Autodesk Inventor part; units mm, degrees
ref_plane "YZ Plane" through (0, 0, 0) normal (1, 0, 0) x (0, 1, 0)
ref_plane "XZ Plane" through (0, 0, 0) normal (0, 1, 0) x (-1, 0, 0)
ref_plane "XY Plane" through (0, 0, 0) normal (0, 0, 1) x (1, 0, 0)
sketch "Sketch1" plane through (0, 0, 0) normal (0, 0, 1) x (1, 0, 0)
  line L0 (0, 0) -> (0, 152.8559)
  line L1 (0, 152.8559) -> (-25, 138.4222)
  line L2 (-25, 138.4222) -> (-25, 0)
  line L3 (-25, 0) -> (25, 0)
  line L4 (25, 0) -> (25, 138.4222)
  line L5 (25, 138.4222) -> (0, 152.8559)
  dimension "d0" = 152.8559
  dimension "d1" = 60
  dimension "d2" = 60
  dimension "d3" = 50
extrude "Extrusion1" add sketch "Sketch1" along normal blind 10
sketch "Sketch2" plane through (0, 0, 0) normal (0, 0, -1) x (-1, 0, 0)
  line L0 (0, 152.8559) -> (25, 138.4222)
  line L1 (-25, 138.4222) -> (0, 152.8559)
  line L2 (25, 0) -> (-25, 0)
  line L3 (-25, 0) -> (25, 0)
  line L4 (25, 0) -> (25, 10)
  line L5 (25, 10) -> (-25, 10)
  line L6 (-25, 10) -> (-25, 0)
  line L7 (25, 138.4222) -> (25, 0) construction
  line L8 (-25, 0) -> (-25, 138.4222) construction
  line L9 (-25, 126.8751) -> (0, 141.3089)
  line L10 (0, 141.3089) -> (25, 126.8751)
  line L11 (25, 138.4222) -> (25, 0)
  line L12 (-25, 126.8751) -> (-25, 138.4222)
  line L13 (0, 152.8559) -> (25, 138.4222)
  line L14 (25, 126.8751) -> (25, 138.4222)
  point P0 (0, 0)
  dimension "d6" = 10
  dimension "d7" = 10
extrude "Extrusion2" add sketch "Sketch2" along normal blind 50
sketch "Sketch3" plane through (0, 141.3089, -50) normal (-0.5, -0.8660254, 0) x (0.8660254, -0.5, 0)
  circle A0 centre (14.4338, 25) radius 2.5
  line L0 (28.8675, 50) -> (28.8675, 0)
  line L1 (28.8675, 0) -> (0, 0)
  point P0 (70.6545, 50)
  point P1 (14.4338, 0)
  point P2 (28.8675, 25)
  dimension "d10" = 5
extrude "Extrusion3" cut sketch "Sketch3" against normal through all
sketch "Sketch4" plane through (-25, 126.8751, -50) normal (0.5, -0.8660254, 0) x (0.8660254, 0.5, 0)
  line L0 (0, 50) -> (0, 0)
  line L1 (28.8675, 0) -> (0, 0)
  circle A0 centre (14.4338, 25) radius 2.5
  point P0 (-41.7869, 50)
  point P1 (14.4338, 0)
  point P2 (0, 25)
  dimension "d13" = 5
extrude "Extrusion4" cut sketch "Sketch4" against normal through all
sketch "Sketch5" plane through (-25, 10, 0) normal (0, 1, 0) x (1, 0, 0)
  line L0 (0, 0) -> (0, 50)
  line L1 (0, 50) -> (50, 50)
  circle A0 centre (25, 25) radius 2.5
  point P0 (25, 0)
  point P1 (25, 50)
  point P2 (0, 25)
  dimension "d16" = 5
extrude "Extrusion5" cut sketch "Sketch5" against normal through all
sketch "Sketch6" plane through (0, 0, 10) normal (0, 0, 1) x (1, 0, 0)
  circle A0 centre (0, 76.428) radius 6
  line L0 (-25, 138.4222) -> (0, 152.8559) construction
  line L1 (0, 152.8559) -> (0, 0) construction
  circle A1 centre (0, 69.428) radius 1.5 construction
  circle A2 centre (15.5, 69.428) radius 1.5
  circle A3 centre (7.75, 82.8513) radius 1.5
  circle A4 centre (-7.75, 82.8513) radius 1.5
  circle A5 centre (-15.5, 69.428) radius 1.5
  circle A6 centre (-7.75, 56.0046) radius 1.5
  circle A7 centre (7.75, 56.0046) radius 1.5
  point P0 (0, 76.428)
  dimension "d19" = 12
  dimension "d22" = 3
  dimension "d23" = 7
  dimension "d24" = 3
  dimension "d25" = 15.5
  dimension "d28" = 360
extrude "Extrusion6" cut sketch "Sketch6" against normal through all
sketch "Sketch7" plane through (0, 0, 0) normal (0, 0, -1) x (-1, 0, 0)
  circle A0 centre (-7.75, 56.0046) radius 1.5
  circle A1 centre (15.5, 69.428) radius 1.5
  circle A2 centre (-7.75, 82.8513) radius 1.5
  circle A3 centre (-15.5, 69.428) radius 1.5
  circle A4 centre (7.75, 82.8513) radius 1.5
  circle A5 centre (7.75, 56.0046) radius 1.5
  circle A6 centre (0, 76.428) radius 6
  line L0 (-25, 10) -> (25, 10)
  line L1 (25, 126.8751) -> (25, 10)
  line L2 (25, 126.8751) -> (0, 141.3089)
  line L3 (0, 141.3089) -> (-25, 126.8751)
  line L4 (-25, 10) -> (-25, 126.8751)
  circle A7 centre (0, 69.428) radius 20
  point P0 (0, 0)
  dimension "d32" = 40
extrude "Extrusion7" cut sketch "Sketch7" against normal blind 5 contours A0 | A1 | A2 | A3 | A4 | A5 | A6 | A7
sketch "Sketch8" plane through (0, 0, 10) normal (0, 0, 1) x (1, 0, 0)
  circle A0 centre (15.5, 69.428) radius 1.5
  circle A1 centre (0, 69.428) radius 1.5
  line L0 (-25, 0) -> (25, 0)
  circle A2 centre (15.5, 69.428) radius 4
  circle A3 centre (7.75, 82.8513) radius 4
  circle A4 centre (-7.75, 82.8513) radius 4
  circle A5 centre (-15.5, 69.428) radius 4
  circle A6 centre (-7.75, 56.0046) radius 4
  circle A7 centre (7.75, 56.0046) radius 4
  point P0 (0, 0)
  point P1 (0, 0)
  dimension "d35" = 3
  dimension "d36" = 8
  dimension "d39" = 360
extrude "Extrusion8" cut sketch "Sketch8" against normal blind 3 contours A0 | A2 | A3 | A4 | A5 | A6 | A7
properties part number "BO12" material "ABS Plastic"
Can you work these out from the model? Positions are in its coordinate system, mm. A direction names the side the tool comes from. Coordinates: 2 decimals unless noted, no trailing zeros. Order: outer loops, then holes, each group sorted by start corner. A loop starts at its lowest first (then second) coordinate and runs counter-clockwise, first axis right, second up.
1. If we section it at B-B (x = 7.75): Please give me the cut outline in (y, z).
2. If we section it at D-D (z = -25): Please give me the cut outline in (x, y), then the cut area to 3 significant figures.
3. For faces 4 (the face through (-15.6, 67.7, 7)), 5 (the face through (-8.08, 54.54, 6.01)), 6 (the face through (-25, 64, 2)), 7 (the face through (0, 10, -19)), 8 (the face through (-15.1, 132.59, -24.65)), which set-ups out of +Z, -Z, +X, -X, +Y, -Y let a thin tool reach every point of the face, with its end or its side?
4. If we section it at A-A (z = -43.5): Please give me the cut outline in (x, y).
5. I need wall thicknesses on line 1 (Y direction, x = 7, z = 6); line 2 (Z direction, x = -12, y = 108.5); line 3 (Z direction, x = 17, y = 76). Which ranges of each line are inside material? Lowest first, please.
6. I'm going to push flat-ended pins straight in: pin 1 (4 mm diameter, centred on x = 7.75, y = 56, fed in from +Z); pin 2 (7 mm diameter, centred on x = 0, y = 76.428, fed in from -Z); pin 3 (5 mm diameter, centred on x = 15.5, y = 69.428, fed in from -Z); pin 4 (25 mm diameter, centred on x = -11.5, y = 43, fed in from -Z). Where does each tip first touch, or does it pass through?
7. Thinking about a two-plate mould opening in Y: for faces 1 (the face through (-12.325, 145.74, -20.42)), 2 (the face through (0, 0, -20)), 3 (the face through (9.897, 135.595, -24.65)), which applies, +Y half, -Y half, draft (parallel to the pull), parting line (faces both ways), or undercut?
8. If we section it at C-C (y = 17.5): Please give me the cut outline in (x, z), then the cut area to 3 significant figures.
Entries:
1. outline: (0, -50) - (10, -50) - (10, 0) - (50.99, 0) - (50.99, 5) - (54.5, 5) - (54.5, 7) - (52, 7) - (52, 10) - (0, 10) - close; (57.5, 5) - (81.35, 5) - (81.35, 7) - (78.85, 7) - (78.85, 10) - (60, 10) - (60, 7) - (57.5, 7) - close; (84.35, 5) - (87.87, 5) - (87.87, 0) - (136.83, 0) - (136.83, -50) - (148.38, -50) - (148.38, 10) - (86.85, 10) - (86.85, 7) - (84.35, 7) - close
2. outline: (-25, 0) - (-2.5, 0) - (-2.5, 10) - (-25, 10) - close; (-25, 126.88) - (-14.67, 132.84) - (-19.67, 141.5) - (-25, 138.42) - close; (-15.33, 144) - (-10.33, 135.34) - (0, 141.31) - (10.33, 135.34) - (15.33, 144) - (0, 152.86) - close; (2.5, 0) - (25, 0) - (25, 10) - (2.5, 10) - close; (14.67, 132.84) - (25, 126.88) - (25, 138.42) - (19.67, 141.5) - close
2. area: 927 mm2
3. face 4: +Z
3. face 5: +Z, -Z
3. face 6: +Z, -Z, -X, +Y, -Y
3. face 7: -Z, +X, -X
3. face 8: -Z
4. outline: (-25, 0) - (25, 0) - (25, 10) - (-25, 10) - close; (-25, 126.88) - (0, 141.31) - (25, 126.88) - (25, 138.42) - (0, 152.86) - (-25, 138.42) - close
5. line 1: y = 0 to 54.71, 57.3 to 81.55, 84.15 to 148.81
5. line 2: z = 0 to 10
5. line 3: z = 5 to 10
6. pin 1: stops at z = 7
6. pin 2: passes through
6. pin 3: stops at z = 5
6. pin 4: stops at z = 0
7. face 1: +Y half
7. face 2: -Y half
7. face 3: undercut
8. outline: (-25, 0) - (25, 0) - (25, 10) - (-25, 10) - close
8. area: 500 mm2
